The drawing under review shows one solid part. Ordinate dimensions are in mm from its lowest x, y, z. Coordinates: 2 decimals unless noted, no trailing zeros. Loops run counter-clockwise (first coordinate to the right, second up) from the corner with the lowest first, then second, coordinate; pieces in that order, holes last. Notation, with made-up numbers: M 40,0.25 L 56,0.25 A18 cw 56,16.25 Z; hole C 47,61 d6. An arc over 180 degrees is marked long. Use one line per item in the form item = value.
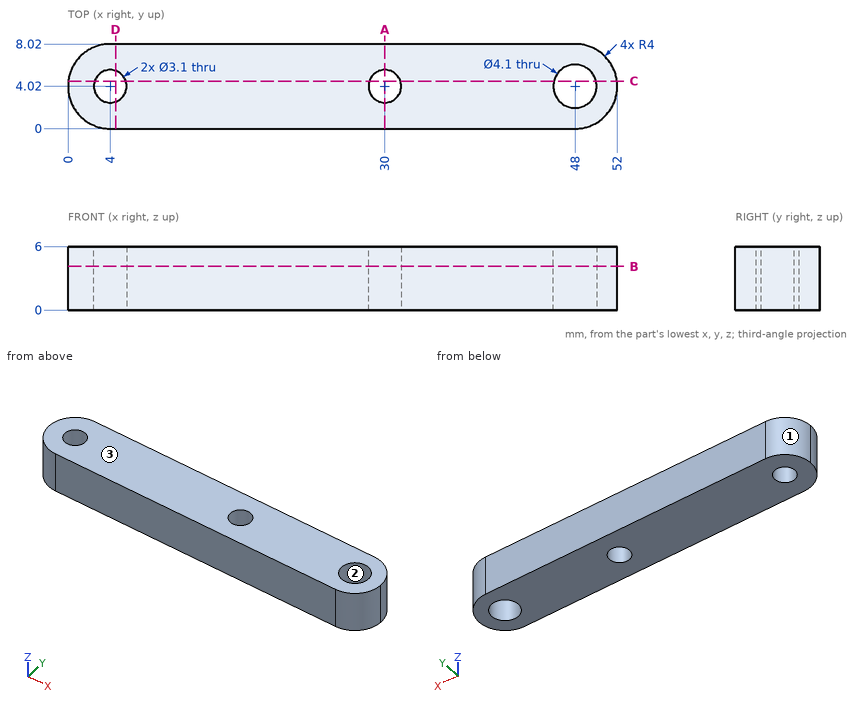
1. Wall thickness on line 1 along X through (y, z) = (4.02, 2.1); line 2 along Y through (x, z) = (30, 4.5); line 3 along X through (y, z) = (3.25, 1.7): over which ranges is each line inside the solid? List them lowest first. Write a range as from..to.
Computed values:
line_1 = 0..2.45, 5.55..28.45, 31.55..45.95, 50.05..52
line_2 = 0..2.47, 5.57..8.02
line_3 = 0.07..2.65, 5.35..28.65, 31.35..46.1, 49.9..51.93
2. Consider section A-A on x = 30. Write out the cut boundary in (y, z).
Computed values:
outline = M 0,0 L 2.47,0 L 2.47,6 L 0,6 Z; M 5.57,0 L 8.02,0 L 8.02,6 L 5.57,6 Z
3. Draft analysis for pull direction X (two halves, no side actions). For the marked faces 1, 2 and 3, state which applies: +X half, -X half, draft (parallel to the pull), parting line (faces both ways), or undercut.
Computed values:
face_1 = -X half
face_2 = undercut
face_3 = draft
4. Consider section C-C on y = 4.5. Write out the cut boundary in (x, z), plus the area to 3 significant figures.
Computed values:
outline = M 0.03,0 L 2.53,0 L 2.53,6 L 0.03,6 Z; M 5.47,0 L 28.53,0 L 28.53,6 L 5.47,6 Z; M 31.47,0 L 46.01,0 L 46.01,6 L 31.47,6 Z; M 49.99,0 L 51.97,0 L 51.97,6 L 49.99,6 Z
area = 252 mm2
5. Consider section B-B on z = 4.15. State how many separate pieces and enclosed holes the cut face has, plus the area to 3 significant figures.
Computed values:
separate_pieces = 1
enclosed_holes = 3
area = 375 mm2
6. Consider section D-D on x = 4.5. Write out the cut boundary in (y, z), plus the area to 3 significant figures.
Computed values:
outline = M 0,0 L 2.55,0 L 2.55,6 L 0,6 Z; M 5.49,0 L 8.02,0 L 8.02,6 L 5.49,6 Z
area = 30.5 mm2
